Geometry: final body of the model. Coordinates: model frame, mm. Face numbers are marked on the shaded views. A direction names the side the tool comes from. Give positions to 0.01 mm unless a question says otherwise; leave off trailing zeros. Write each loop counter-clockwise with the first axis right and the second up, starting at its lowest first coordinate (ties: lowest second). Pieces come first, ordered by that corner, then holes. Notation, with made-up numbers: (-8, 58.5) - (-1, 58.5) arc R33 ccw to (-1, 86.5) - close; hole circle Ø9 at (54.5, 68.25). An arc over 180 degrees is marked (long way). Use CSV: the item, a comma, the result in double quotes. Start each with the question number.
(1) Section D-D on z = 8.5. Output: boundary loops of the cut face in (x, y).
(2) Section B-B on y = -4.25. Output: boundary loops of the cut face in (x, z).
(3) Section A-A on x = -36. Output: boundary loops of the cut face in (y, z).
(4) Line query: probe 1 along X at (y, z) = (-5.25, 5); probe 2 along X at (y, z) = (-1, 5); probe 3 along Z at (x, y) = (36, -2.5). Output: solid intervals per line, ascending. Write a range as [from, to].
(5) Section C-C on z = 5. Output: boundary loops of the cut face in (x, y).
(6) Reachability of the marked faces 1 and 2 from +Z, -Z, +X, -X, +Y, -Y: full face, straight path, thin tool, end or side. Return the list, or none.
from build123d import *

# Parameters (mm, degrees)
BOSS_EXTRUDE1_DEPTH = 10
FILLET1_R           = 2.5
CUT_EXTRUDE1_REACH  = 22
SKETCH2_R           = 2.5


with BuildPart() as part:
    # Sketch1 → Boss-Extrude1 (new body)
    with BuildSketch(Plane.XY):
        Polygon((0, 6.5), (0, 0), (31, 0), (31, -13.5), (41, -13.5), (41, 6.5), align=None)
        Polygon((-31, 0), (0, 0), (0, 6.5), (-41, 6.5), (-41, -13.5), (-31, -13.5), align=None)
    extrude(amount=BOSS_EXTRUDE1_DEPTH)

    # Fillet1
    fillet1_edges = [part.edges().sort_by_distance(p)[0] for p in [
        (31, 0, 5),
        (-31, 0, 5),
    ]]
    fillet(fillet1_edges, radius=FILLET1_R)

    # Sketch2 → Cut-Extrude1 (cut, up to next)
    with BuildSketch(Plane(origin=(0, 6.5, 0), x_dir=(1, 0, 0), z_dir=(0, 1, 0)), mode=Mode.PRIVATE) as cut_extrude1_sk1:
        with Locations((-36, -5)):
            Circle(SKETCH2_R)
    cut_extrude1_tool1 = extrude(cut_extrude1_sk1.sketch, amount=-CUT_EXTRUDE1_REACH, mode=Mode.PRIVATE) & part.part
    add(cut_extrude1_tool1.solids().sort_by_distance((-36, 6.5, 5))[0], mode=Mode.SUBTRACT)
    # Sketch2 → Cut-Extrude1 (cut, up to next)
    with BuildSketch(Plane(origin=(0, 6.5, 0), x_dir=(1, 0, 0), z_dir=(0, 1, 0)), mode=Mode.PRIVATE) as cut_extrude1_sk2:
        with Locations((36, -5)):
            Circle(SKETCH2_R)
    cut_extrude1_tool2 = extrude(cut_extrude1_sk2.sketch, amount=-CUT_EXTRUDE1_REACH, mode=Mode.PRIVATE) & part.part
    add(cut_extrude1_tool2.solids().sort_by_distance((36, 6.5, 5))[0], mode=Mode.SUBTRACT)


solid = part.part
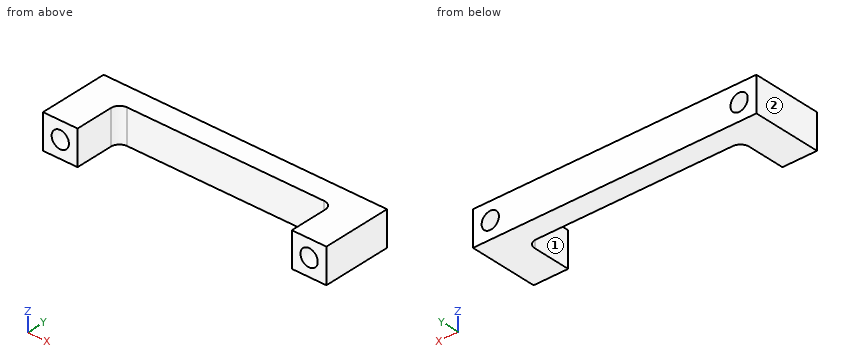
Check values:
1,outline,"(-41, -13.5) - (-31, -13.5) - (-31, -2.5) arc R2.5 cw to (-28.5, 0) - (28.5, 0) arc R2.5 cw to (31, -2.5) - (31, -13.5) - (41, -13.5) - (41, 6.5) - (-41, 6.5) - close"
2,outline,"(-41, 0) - (-31, 0) - (-31, 10) - (-41, 10) - close; (31, 0) - (41, 0) - (41, 10) - (31, 10) - close; hole circle Ø5 at (-36, 5); hole circle Ø5 at (36, 5)"
3,outline,"(-13.5, 0) - (6.5, 0) - (6.5, 2.5) - (-13.5, 2.5) - close; (-13.5, 7.5) - (6.5, 7.5) - (6.5, 10) - (-13.5, 10) - close"
4,probe 1,"x = [-41, -38.5], [-33.5, -31], [31, 33.5], [38.5, 41]"
4,probe 2,"x = [-41, -38.5], [-33.5, -30.5], [30.5, 33.5], [38.5, 41]"
4,probe 3,"z = [0, 2.5], [7.5, 10]"
5,outline,"(-41, -13.5) - (-38.5, -13.5) - (-38.5, 6.5) - (-41, 6.5) - close; (-33.5, -13.5) - (-31, -13.5) - (-31, -2.5) arc R2.5 cw to (-28.5, 0) - (28.5, 0) arc R2.5 cw to (31, -2.5) - (31, -13.5) - (33.5, -13.5) - (33.5, 6.5) - (-33.5, 6.5) - close; (38.5, -13.5) - (41, -13.5) - (41, 6.5) - (38.5, 6.5) - close"
6,face 1,"+Z, -Z, -Y"
6,face 2,"+Z, -Z, -X, +Y, -Y"
